Input: part model. Units: mm. Frame: model coordinates. Face numbers are marked on the shaded views. A direction names the side the tool comes from. Round coordinates to 2 decimals unless told otherwise and drop trailing zeros. Loops run counter-clockwise (first coordinate to the right, second up) from the corner with the lowest first, then second, coordinate; pieces in that order, holes last. Notation, with made-up numbers: (-17.75, -33) -> (15.25, -33) arc R25 cw to (15.25, -11) -> close; hole circle Ø11 at (-37.5, 66.25). An arc over 180 degrees is marked (long way). Answer in a Markdown table with one row per item. Add a question column.
Q1. Section C-C, the plane y = -29.5. Output: boundary loops of the cut face in (x, z), and give its area (3 significant figures).
Q2. Ray query, L1, parallel to Y at x = 15, z = 3.5; L2, parallel to Z at x = 5, y = -32.5; L3, parallel to X at y = -19, z = 31. Return the intervals inside material, ascending. Write a range as from..to.
Q3. Section A-A, the plane y = -19.05. Output: boundary loops of the cut face in (x, z).
Q4. Section B-B, the plane x = -124. Output: boundary loops of the cut face in (y, z) (3 decimals).
Q5. Pin query (flat end, axial travel): pin 1 (21.5 mm diameter, centred on x = -112.8, z = 13.38, fed in from -Y); pin 2 (2 mm diameter, centred on x = -115.5, z = 3, fed in from -Y); pin 3 (20.5 mm diameter, centred on x = -52, y = -21.5, fed in from -Z); pin 4 (2 mm diameter, centred on x = -64.5, z = 5, fed in from +Y). Return the tip coordinate at first contact, or that it passes through.
Q6. Section D-D, the plane y = -6. Output: boundary loops of the cut face in (x, z).
Q7. Reachability of the marked faces 1 and 2 from +Z, -Z, +X, -X, +Y, -Y: full face, straight path, thin tool, end or side. Return the list, or none.
```python
from build123d import *

# Parameters (mm, degrees)
F1_DEPTH = 190.5
F5_D     = 13.49248
F6_D     = 13.49248


with BuildPart() as f1:
    # F0 (on Right) → F1 (new body)
    with BuildSketch(Plane.YZ):
        with BuildLine():
            Line((-0.1024892145, -7.1891873267), (0, -7.1925527072))
            Line((0, -7.1925527072), (0, 30.9074472928))
            Line((0, 30.9074472928), (-38.1, 30.9074472928))
            ThreePointArc((-38.1, 30.9074472928), (-37.1700640303, 28.6623832625), (-34.925, 27.7324472928))
            Line((-34.925, 27.7324472928), (-9.5232896904, 27.7324472928))
            ThreePointArc((-9.5232896904, 27.7324472928), (-5.0331616299, 25.8725753533), (-3.1732896904, 21.3824472928))
            Line((-3.1732896904, 21.3824472928), (-3.1732896904, -4.0158976363))
            ThreePointArc((-3.1732896904, -4.0158976363), (-2.2798964147, -6.223814246), (-0.1024892145, -7.1891873267))
        make_face()
    extrude(amount=F1_DEPTH)


with BuildPart() as f1_1:
    # F2: moved
    add(f1.part.moved(Location((-137.16, 0, 1.524))))

    # F5 (through all)
    with Locations(Plane.XY.offset(32.4314472928)):
        with Locations((-112.8014, -19.05)):
            Hole(F5_D / 2)

    # F6 (through all)
    with Locations(Plane.XZ.offset(3.1732896904)):
        with Locations((-112.8014, 13.3831023637)):
            Hole(F6_D / 2)


solid = f1_1.part
```
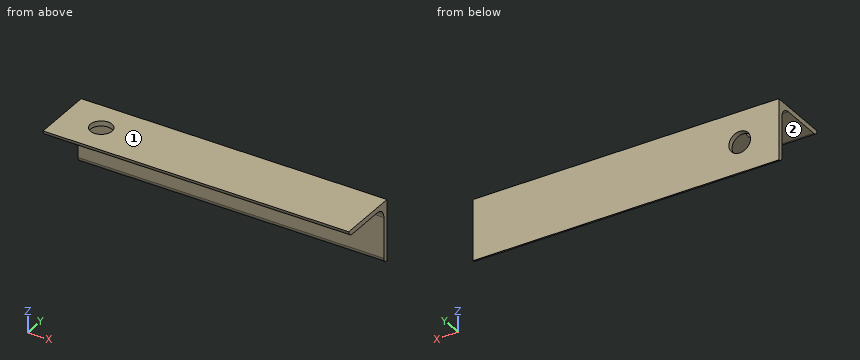
Answer block:
| question | item | result |
|---|---|---|
| 1 | outline | (-137.16, 29.26) -> (53.34, 29.26) -> (53.34, 32.43) -> (-137.16, 32.43) -> close |
| 1 | area | 605 mm^2 |
| 2 | L1 | -3.17..0 |
| 2 | L2 | 29.26..32.43 |
| 2 | L3 | -137.16..-119.55, -106.06..53.34 |
| 3 | outline | (-137.16, 29.26) -> (-119.55, 29.26) -> (-119.55, 32.43) -> (-137.16, 32.43) -> close; (-106.06, 29.26) -> (53.34, 29.26) -> (53.34, 32.43) -> (-106.06, 32.43) -> close |
| 4 | outline | (-38.1, 32.431) arc R3.175 ccw to (-34.925, 29.256) -> (-9.523, 29.256) arc R6.35 cw to (-3.173, 22.906) -> (-3.173, -2.492) arc R3.175 ccw to (-0.102, -5.665) -> (0, -5.669) -> (0, 32.431) -> close |
| 5 | pin 1 | y = -3.29 |
| 5 | pin 2 | y = -3.17 |
| 5 | pin 3 | z = 29.26 |
| 5 | pin 4 | y = 0 |
| 6 | outline | (-137.16, 28.19) -> (53.34, 28.19) -> (53.34, 32.43) -> (-137.16, 32.43) -> close |
| 7 | face 1 | +Z, +X, -X, +Y, -Y |
| 7 | face 2 | -Z, +X, -X, -Y |
